Autodesk Inventor part; units mm, degrees
ref_plane "Work Plane1" through (11.2, 0, 23) normal (0, -1, 0) x (1, 0, 0)
ref_plane "Work Plane2" through (0, -6.2, 3) normal (-1, 0, 0) x (0, 0, 1)
ref_plane "YZ Plane" through (0, 0, 0) normal (1, 0, 0) x (0, 1, 0)
sketch "Sketch1" plane through (0, 0, 0) normal (0, 0, 1) x (1, 0, 0)
  line L0 (0, 6.93) -> (0, -6.93) construction
  line L1 (-13.93, 0) -> (13.93, 0) construction
  line L2 (-9.95, 4.95) -> (9.95, 4.95)
  line L3 (9.95, 4.95) -> (9.95, -4.95)
  line L4 (9.95, -4.95) -> (-9.95, -4.95)
  line L5 (-9.95, -4.95) -> (-9.95, 4.95)
  point P0 (0, 0)
  dimension "d0" = 9.9
  dimension "d1" = 19.9
extrude "Extrusion1" add sketch "Sketch1" along normal blind 3
sketch "Sketch2" plane through (0, 0, 3) normal (0, 0, 1) x (1, 0, 0)
  line L0 (9.95, 4.95) -> (-9.95, 4.95) construction
  line L1 (-9.95, 4.95) -> (-9.95, -4.95) construction
  line L2 (-9.95, -4.95) -> (9.95, -4.95) construction
  line L3 (9.95, -4.95) -> (9.95, 4.95) construction
  line L4 (11.2, 6.2) -> (-11.2, 6.2)
  line L5 (-11.2, 6.2) -> (-11.2, -6.2)
  line L6 (-11.2, -6.2) -> (11.2, -6.2)
  line L7 (11.2, -6.2) -> (11.2, 6.2)
  point P0 (0, 0)
  dimension "d" = 1.25
  dimension "d5" = 1.25
  dimension "d6" = 1.25
  dimension "d7" = 1.25
extrude "Extrusion2" add sketch "Sketch2" along normal blind 20
sketch "Sketch3" plane through (0, 0, 23) normal (0, 0, 1) x (1, 0, 0)
  line L0 (11.2, 6.2) -> (-11.2, 6.2) construction
  line L1 (-11.2, 6.2) -> (-11.2, -6.2) construction
  line L2 (-11.2, -6.2) -> (11.2, -6.2) construction
  line L3 (11.2, -6.2) -> (11.2, 6.2) construction
  line L4 (0, 8.68) -> (0, -8.68) construction
  line L5 (-21, 0) -> (21, 0) construction
  line L6 (15, 6.2) -> (-15, 6.2)
  line L7 (-15, 6.2) -> (-15, -6.2)
  line L8 (-15, -6.2) -> (15, -6.2)
  line L9 (15, -6.2) -> (15, 6.2)
  point P0 (0, 0)
  dimension "d10" = 30
extrude "Extrusion3" add sketch "Sketch3" along normal blind 5
sketch "Sketch4" plane through (0, 0, 28) normal (0, 0, 1) x (1, 0, 0)
  line L0 (0, 17.5) -> (0, -17.5) construction
  line L1 (-21, 0) -> (21, 0) construction
  line L2 (15, 6.2) -> (-15, 6.2) construction
  line L3 (-15, 6.2) -> (-15, -6.2) construction
  line L4 (-15, -6.2) -> (15, -6.2) construction
  line L5 (15, -6.2) -> (15, 6.2) construction
  line L6 (12.5, 12.5) -> (-12.5, 12.5)
  line L7 (-12.5, 12.5) -> (-12.5, -12.5)
  line L8 (-12.5, -12.5) -> (12.5, -12.5)
  line L9 (12.5, -12.5) -> (12.5, 12.5)
  point P0 (0, 0)
  dimension "d13" = 25
  dimension "d14" = 25
extrude "Extrusion4" cut sketch "Sketch4" against normal blind 2.5
sketch "Sketch5" plane through (0, 0, 25.5) normal (0, 0, 1) x (1, 0, 0)
  point P0 (0, 0)
  point P1 (0, 0)
hole "Hole1" at (0, 0, 25.5) direction (0, 0, -1) diameter 3.242 depth 10 tip angle 118
sketch "Sketch6" plane through (-11.2, -6.2, 3) normal (0, -1, 0) x (1, 0, 0)
  line L0 (-1.3, 22.5) -> (-1.3, 25) construction
  line L1 (-3.8, 25) -> (-1.3, 25) construction
  line L2 (-3.8, 20) -> (-3.8, 25) construction
  line L3 (-3.8, 20) -> (0, 20) construction
  line L4 (0, 0) -> (0, 20) construction
  line L5 (0, 0) -> (22.4, 0) construction
  line L6 (22.4, 0) -> (22.4, 20) construction
  line L7 (22.4, 20) -> (26.2, 20) construction
  line L8 (26.2, 20) -> (26.2, 25) construction
  line L9 (23.7, 25) -> (26.2, 25) construction
  line L10 (23.7, 25) -> (23.7, 22.5) construction
  line L11 (23.7, 22.5) -> (-1.3, 22.5) construction
  line L12 (11.2, 30.6) -> (11.2, -8.6) construction
  line L13 (0, 0) -> (22.4, 0)
  line L14 (3.2, 0) -> (11.2, 0)
  arc A0 (6.2, 3) -> (3.2, 0) centre (6.2, 0) ccw
  line L15 (6.2, 3) -> (11.2, 3)
  line L16 (19.2, 0) -> (11.2, 0)
  arc A1 (19.2, 0) -> (16.2, 3) centre (16.2, 0) ccw
  line L17 (16.2, 3) -> (11.2, 3)
  point P0 (11.2, -3)
  dimension "d24" = 8
  dimension "r" = 3
  dimension "d28" = 3
extrude "Extrusion5" add sketch "Sketch6" along normal blind 2
sketch "Sketch7" plane through (-11.2, -8.2, 3) normal (0, -1, 0) x (1, 0, 0)
  line L0 (3.2, 0) -> (19.2, 0) construction
  arc A0 (19.2, 0) -> (16.2, 3) centre (16.2, 0) ccw construction
  line L1 (16.2, 3) -> (6.2, 3) construction
  arc A1 (6.2, 3) -> (3.2, 0) centre (6.2, 0) ccw construction
  line L2 (2.2, 0) -> (20.2, 0) construction
  arc A2 (6.2, 4) -> (2.2, 0) centre (6.2, 0) ccw
  arc A3 (20.2, 0) -> (16.2, 4) centre (16.2, 0) ccw
  line L3 (6.2, 4) -> (16.2, 4)
  line L4 (2.2, 0) -> (20.2, 0)
  point P0 (11.2, -3)
  dimension "d33" = 1
  dimension "a" = 1
extrude "Extrusion6" add sketch "Sketch7" along normal blind 1
ref_plane "Work Plane1" through (11.2, 0, 23) normal (0, -1, 0) x (1, 0, 0)
ref_plane "Work Plane2" through (0, -6.2, 3) normal (-1, 0, 0) x (0, 0, 1)
mirror "Mirror1" about plane through (11.2, 0, 23) normal (0, -1, 0) of "Extrusion5", "Extrusion6"
sketch "Sketch8" plane through (-11.2, -6.2, 3) normal (-1, 0, 0) x (0, 0, 1)
  line L0 (0, 12.4) -> (0, 0) construction
  line L1 (0, 0) -> (20, 0) construction
  line L2 (20, 12.4) -> (20, 0) construction
  line L3 (0, 12.4) -> (20, 12.4) construction
  line L4 (30.6, 6.2) -> (-8.6, 6.2) construction
  line L5 (15, 10.2) -> (15, 6.2)
  arc A0 (16, 9.2) -> (15, 10.2) centre (15, 9.2) ccw
  line L6 (15, 9.2) -> (16, 9.2) construction
  line L7 (15, 9.2) -> (15, 10.2) construction
  line L8 (16, 9.2) -> (16, 6.2)
  line L9 (15, 2.2) -> (15, 6.2)
  arc A1 (15, 2.2) -> (16, 3.2) centre (15, 3.2) ccw
  line L10 (16, 3.2) -> (16, 6.2)
  point P0 (-3, 6.2)
  dimension "d37" = 4
  dimension "d38" = 90
  dimension "radius" = 1
  dimension "d40" = 15
extrude "Extrusion7" add sketch "Sketch8" along normal blind 2
sketch "Sketch9" plane through (-13.2, -6.2, 3) normal (-1, 0, 0) x (0, 0, 1)
  line L0 (15, 10.2) -> (15, 2.2) construction
  arc A0 (15, 2.2) -> (16, 3.2) centre (15, 3.2) ccw construction
  line L1 (16, 3.2) -> (16, 9.2) construction
  arc A1 (16, 9.2) -> (15, 10.2) centre (15, 9.2) ccw construction
  line L2 (15, 11.2) -> (15, 1.2)
  arc A2 (17, 9.2) -> (15, 11.2) centre (15, 9.2) ccw
  arc A3 (15, 1.2) -> (17, 3.2) centre (15, 3.2) ccw
  line L3 (17, 9.2) -> (17, 3.2)
  line L4 (15, 10.2) -> (15, 2.2)
  point P0 (-3, 6.2)
  dimension "d44" = 1
  dimension "d45" = 1
  dimension "d46" = 90
extrude "Extrusion8" add sketch "Sketch9" along normal blind 1
fillet "Fillet1" radius 0.25 5 edges at (-12.2, 4, 18) (-13.7, 5, 18) (-13.7, -5, 18) (-12.2, -4, 18) (-14.2, 0, 18)
mirror "Mirror2" about plane through (0, -6.2, 3) normal (-1, 0, 0) of "Extrusion7", "Extrusion8", "Fillet1"
equation "\"d5\" = d"
equation "\"d6\" = d"
equation "\"d7\" = d"
equation "\"d28\" = r"
equation "\"d33\" = a"
properties part number "Sample-cuvette-clamp-20mm-V4"
Can you work these out from the model? Positions are in its coordinate system, mm. A direction names the side the tool comes from. Give positions to 0.01 mm unless a question says otherwise; leave off trailing zeros. Order: outer loops, then holes, each group sorted by start corner. A loop starts at its lowest first (then second) coordinate and runs counter-clockwise, first axis right, second up. Notation, with made-up numbers: M 65,16 L 89,16 A19 cw 89,53 Z; hole C -21,-8.75 d2. An arc over 180 degrees is marked long. Use one line per item in the form item = value. Start each with the question number.
Item 1: We'd pull the mould along X, two halves only. Please class faces 1 (the flat face through (0, 9, 7)), 2 (the flat face through (12, 0, 19)), 3 (the cylindrical face through (-7.14, -7.19, 5.1)): +X half, -X half, draft (parallel to the pull), parting line (faces both ways), or undercut.
Item 2: If I drill on line 1 along Y through (x, z) = (0, 21.25); line 2 along X through (y, z) = (0, 21.5); line 3 along Y through (x, z) = (-9, 9.75), over which ranges is the centre line in solid material (lowest first)?
Item 3: If we section it at D-D (z = 11): Write out the boundary of the cut face in (x, y), then the cut area to 3 significant figures.
Item 4: Will these pins go through, and if not, where does the flat tip stop? pin 1 Ø3 at (x, y) = (13, -1) entering from -Z; pin 2 Ø12.5 at (x, z) = (-1, 10.5) entering from -Y; pin 3 Ø10 at (y, z) = (0.5, 10.5) entering from +X; pin 4 Ø4 at (x, z) = (0, 10.5) entering from -Y.
Item 5: If we section it at C-C (x = 2): Write out the boundary of the cut face in (y, z), then the cut area to 3 significant figures.
Item 6: If we section it at A-A (z = 26): Write out the boundary of the cut face in (x, y).
Item 7: For faces 4 (the cylindrical face through (7.1, -7.19, 5.14)), 5 (the flat face through (14.2, 0, 19)), 6 (the cylindrical face through (13.693, 4.294, 19.525)), which set-ups out of +Z, -Z, +X, -X, +Y, -Y let a thin tool reach every point of the face, with its end or its side?
Outcome:
q1.face_1 = draft
q1.face_2 = undercut
q1.face_3 = -X half
q2.line_1 = -6.2 to -1.62, 1.62 to 6.2
q2.line_2 = -11.2 to -1.62, 1.62 to 11.2
q2.line_3 = -6.2 to 6.2
q3.outline = M -11.2,-6.2 L 11.2,-6.2 L 11.2,6.2 L -11.2,6.2 Z
q3.area = 278 mm2
q4.pin_1 = 18
q4.pin_2 = -9.2
q4.pin_3 = 11.2
q4.pin_4 = -6.2
q5.outline = M -9.2,3 L -4.95,3 L -4.95,0 L 4.95,0 L 4.95,3 L 9.2,3 L 9.2,7 L 8.2,7 L 8.2,6 L 6.2,6 L 6.2,25.5 L -6.2,25.5 L -6.2,6 L -8.2,6 L -8.2,7 L -9.2,7 Z
q5.area = 329 mm2
q6.outline = M -15,-6.2 L -12.5,-6.2 L -12.5,6.2 L -15,6.2 Z; M 12.5,-6.2 L 15,-6.2 L 15,6.2 L 12.5,6.2 Z
q7.face_4 = +Z, +X
q7.face_5 = -Z, +X, +Y, -Y
q7.face_6 = +X, +Y
